```python
from build123d import *

# Parameters (mm, degrees)
CYLINDER008_R     = 17.5
CYLINDER008_DEPTH = 4
CYLINDER007_R     = 29.17
CYLINDER007_DEPTH = 4


with BuildPart() as cylinder008:
    # Cylinder008 → Cylinder008 (new body)
    with BuildSketch(Plane.XY.offset(45)):
        Circle(CYLINDER008_R)
    extrude(amount=CYLINDER008_DEPTH)


with BuildPart() as cut007:
    # Cylinder007 → Cylinder007 (new body)
    with BuildSketch(Plane.XY.offset(45)):
        Circle(CYLINDER007_R)
    extrude(amount=CYLINDER007_DEPTH)

    # Cut007: cut Cylinder008
    add(cylinder008.part, mode=Mode.SUBTRACT)


solid = cut007.part
```
The listing builds one solid part. Answer for the finished solid, in the listing's coordinates (mm). Round coordinates to 2 decimals unless told otherwise and drop trailing zeros. Loops run counter-clockwise (first coordinate to the right, second up) from the corner with the lowest first, then second, coordinate; pieces in that order, holes last. Notation, with made-up numbers: (37, 12) -> (46, 12) arc R17 cw to (46, 31) -> close; hole circle Ø11 at (49, 16.25). An arc over 180 degrees is marked (long way). Use one line per item in the form item = value.
1. The part is cut by section C-C on z = 48.3. Determine the outline of the cut face in (x, y), and give its area (3 significant figures).
Answer key:
outline = circle Ø58.34 at (0, 0); hole circle Ø35 at (0, 0)
area = 1,710 mm²
2. For a pull along X with two mould halves and no side action, classify faces 1 (the flat face through (13, -13, 49)), 2 (the cylindrical face through (27.823, 8.762, 46.972)), 3 (the cylindrical face through (-13.887, -10.648, 46.972)) as released by +X, released by -X, zero draft, split by the parting line, or undercut.
Answer key:
face_1 = zero draft
face_2 = split by the parting line
face_3 = undercut
3. A flat-ended cylindrical pin translates along its axis: pin 1 Ø1.5 at (y, z) = (7, 46) entering from -X. Find the tip coordinate at first contact, or state that the pin passes through.
Answer key:
pin_1 = -28.49
4. The part is cut by section D-D on y = 19. Determine the outline of the cut face in (x, z), and give its area (3 significant figures).
Answer key:
outline = (-22.13, 45) -> (22.13, 45) -> (22.13, 49) -> (-22.13, 49) -> close
area = 177 mm²
5. The part is cut by section A-A on x = 0. Determine the outline of the cut face in (y, z), and give its area (3 significant figures).
Answer key:
outline = (-29.17, 45) -> (-17.5, 45) -> (-17.5, 49) -> (-29.17, 49) -> close; (17.5, 45) -> (29.17, 45) -> (29.17, 49) -> (17.5, 49) -> close
area = 93.4 mm²
6. Find the intervals of material crossed by probe 1 along Y at (x, z) = (0, 46.25); probe 2 along X at (y, z) = (-5.5, 46.3); probe 3 along Y at (x, z) = (9.5, 47.6), in increasing order. Write a range as [from, to].
Answer key:
probe_1 = [-29.17, -17.5], [17.5, 29.17]
probe_2 = [-28.65, -16.61], [16.61, 28.65]
probe_3 = [-27.58, -14.7], [14.7, 27.58]
